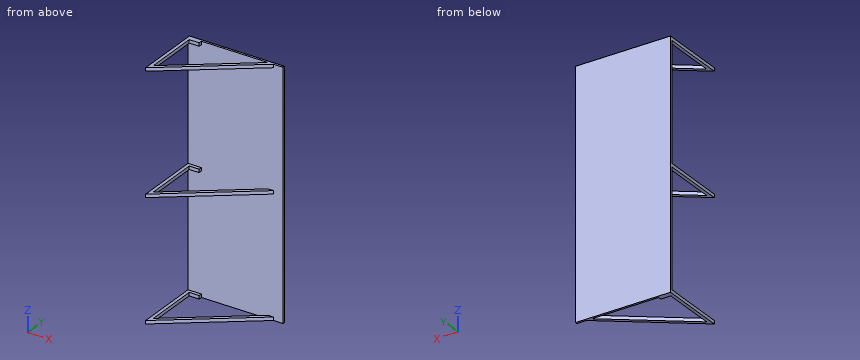
from build123d import *

# Parameters (mm, degrees)
BOSS_EXTRUDE1_DEPTH = 1874.774
SKETCH2_W           = 899.287
SKETCH2_H           = 492.125
CUT_EXTRUDE1_DEPTH  = 731.25


with BuildPart() as part:
    # Sketch1 → Boss-Extrude1 (new body)
    with BuildSketch(Plane.XY):
        Polygon((730.25, 492.125), (656.817236389, 492.125), (0, 0), (0, 508), (730.25, 508), align=None)
        Polygon((101.981819436, 492.125), (101.981819436, 466.725), (25.4, 466.725), (25.4, 50.769813509), (614.457036031, 492.125), align=None, mode=Mode.SUBTRACT)
    extrude(amount=BOSS_EXTRUDE1_DEPTH)

    # Sketch2 → Cut-Extrude1 (cut, through all)
    with BuildSketch(Plane(origin=(730.25, 0, 0), x_dir=(0, 0, -1), z_dir=(1, 0, 0))):
        with Locations((-1399.7305, 246.0625)):
            Rectangle(SKETCH2_W, SKETCH2_H)
        with Locations((-475.0435, 246.0625)):
            Rectangle(SKETCH2_W, SKETCH2_H)
    extrude(amount=-CUT_EXTRUDE1_DEPTH, mode=Mode.SUBTRACT)


solid = part.part
Model file for the job. Use its own axes, mm. Give positions to 0.01 mm unless a question says otherwise; leave off trailing zeros. Loops run counter-clockwise (first coordinate to the right, second up) from the corner with the lowest first, then second, coordinate; pieces in that order, holes last.
1) Saw through at C-C (z = 1098). Write the cut outline in (x, y) (3 decimals).
2) Wall check: line 1 (Y direction, x = 479.5, z = 1502) (3 decimals). Give the ranges that are in metal, low to high.
3) Saw through at B-B (x = 381). Write the cut outline in (y, z) (3 decimals).
4) Flat gauge pins, fed straight in: pin 1 Ø7.5 at (y, z) = (316.5, 934) entering from +X; pin 2 Ø7.5 at (y, z) = (482, 935.5) entering from +X; pin 3 Ø1 at (x, z) = (115.5, 1565) entering from -Y (3 decimals). Where does each tip first touch, or does it go through?
5) Saw through at A-A (y = 227.5). Write the cut outline in (x, z), plus the area to 3 significant figures.
6) Saw through at D-D (x = 676.5). Write the cut outline in (y, z) (3 decimals).
Answer block:
1. outline: (0, 492.125) - (730.25, 492.125) - (730.25, 508) - (0, 508) - close
2. line 1: y = 492.125 to 508
3. outline: (285.467, 0) - (317.206, 0) - (317.206, 25.4) - (285.467, 25.4) - close; (285.467, 924.687) - (317.206, 924.687) - (317.206, 950.087) - (285.467, 950.087) - close; (285.467, 1849.374) - (317.206, 1849.374) - (317.206, 1874.774) - (285.467, 1874.774) - close; (492.125, 0) - (508, 0) - (508, 1874.774) - (492.125, 1874.774) - close
4. pin 1: stops at x = 427.42
4. pin 2: stops at x = 648.31
4. pin 3: stops at y = 492.125
5. outline: (0, 0) - (25.4, 0) - (25.4, 25.4) - (0, 25.4) - close; (0, 924.69) - (25.4, 924.69) - (25.4, 950.09) - (0, 950.09) - close; (0, 1849.37) - (25.4, 1849.37) - (25.4, 1874.77) - (0, 1874.77) - close; (261.27, 0) - (303.63, 0) - (303.63, 25.4) - (261.27, 25.4) - close; (261.27, 924.69) - (303.63, 924.69) - (303.63, 950.09) - (261.27, 950.09) - close; (261.27, 1849.37) - (303.63, 1849.37) - (303.63, 1874.77) - (261.27, 1874.77) - close
5. area: 5,160 mm2
6. outline: (492.125, 0) - (508, 0) - (508, 1874.774) - (492.125, 1874.774) - close
